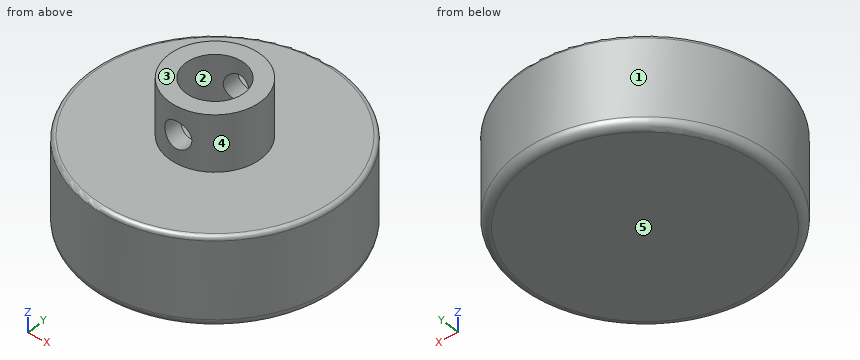
from build123d import *

# Parameters (mm, degrees)
F2_R     = 6.5
F3_DEPTH = 30


with BuildPart() as f1:
    # F0 (on Front) → F1 (revolve)
    with BuildSketch(Plane.XZ):
        with BuildLine():
            Line((-14.1, 0), (-14.1, 27))
            Line((-14.1, 27), (-22.1, 27))
            Line((-22.1, 27), (-22.1, 0))
            Line((-22.1, 0), (-58.77316, 0))
            ThreePointArc((-58.77316, 0), (-60.170035, -0.568658), (-60.772566, -1.95126))
            Line((-60.772566, -1.95126), (-60.772566, -2.403001))
            Line((-60.772566, -2.403001), (-60.772566, -39))
            ThreePointArc((-60.772566, -39), (-59.600994, -41.828427), (-56.772566, -43))
            Line((-56.772566, -43), (-56.4, -43))
            Line((-56.4, -43), (0, -43))
            Line((0, -43), (0, 0))
            Line((0, 0), (-14.1, 0))
        make_face()
    revolve(axis=Axis((0, 0, -21.5), (0, 0, -1)))

    # F2 (on Front) → F3 (cut, symmetric)
    with BuildSketch(Plane.XZ):
        with Locations((0, 13.5)):
            Circle(F2_R)
    extrude(amount=F3_DEPTH, both=True, mode=Mode.SUBTRACT)


solid = f1.part
Read the model definition and answer for the solid it produces. Units are mm, in the model's axes. Face numbers are marked on the shaded views. A direction names the side the tool comes from. Round coordinates to 2 decimals unless told otherwise and drop trailing zeros. Write each loop counter-clockwise with the first axis right and the second up, starting at its lowest first coordinate (ties: lowest second). Pieces come first, ordered by that corner, then holes. Notation, with made-up numbers: M 24,54.5 L 36,54.5 A26 ccw 36,75.5 Z; hole C 47.5,-7 d6. An arc over 180 degrees is marked long. Use a Markdown table: item, result.
1) The part is cut by section A-A (x = 0). Write down the section's boundary in (y, z).
Answers follow:
| item | result |
|---|---|
| outline | M -60.77,-39 A4 ccw -56.77,-43 L 56.77,-43 A4 ccw 60.77,-39 L 60.77,-1.95 A2 ccw 58.77,0 L 22.1,0 L 22.1,7 L 14.1,7 L 14.1,0 L -14.1,0 L -14.1,7 L -22.1,7 L -22.1,0 L -58.77,0 A2 ccw -60.77,-1.95 Z; M -22.1,20 L -14.1,20 L -14.1,27 L -22.1,27 Z; M 14.1,20 L 22.1,20 L 22.1,27 L 14.1,27 Z |
2) A tool of negligible diameter and unlimited length cuts with its end or side. For the marked faces 4 and 5, from which of +Z, -Z, +X, -X, +Y, -Y can it reach the whole face along a straight path? Write none if from no direction.
Answers follow:
| item | result |
|---|---|
| face 4 | +Z |
| face 5 | -Z, +X, -X, +Y, -Y |
3) Flat-ended cylindrical pins translate along their axes: pin 1 (4 mm diameter, centred on x = 44.5, y = 16, fed in from +Z); pin 2 (10 mm diameter, centred on y = 12.5, z = -16.5, fed in from -X); pin 3 (4 mm diameter, centred on x = 3.5, z = -3, fed in from +Y). Find the tip coordinate at first contact, or state that the pin passes through.
Answers follow:
| item | result |
|---|---|
| pin 1 | stops at z = 0 |
| pin 2 | stops at x = -60.31 |
| pin 3 | stops at y = 60.75 |
4) For a pull along X with two mould halves and no side action, classify the marked faces 1, 2 and 3 as pulls with the +X half, pulls with the -X half, needs draft (parallel to the pull), parting line crosses it, or undercut.
Answers follow:
| item | result |
|---|---|
| face 1 | parting line crosses it |
| face 2 | undercut |
| face 3 | needs draft |
5) The part is cut by section B-B (z = 13.5). Write down the section's boundary in (x, y), plus the area to 3 significant figures.
Answers follow:
| item | result |
|---|---|
| outline | M -6.5,-21.12 L -6.5,-12.51 A14.1 cw -6.5,12.51 L -6.5,21.12 A22.1 ccw Z; M 6.5,-21.12 A22.1 ccw 6.5,21.12 L 6.5,12.51 A14.1 cw 6.5,-12.51 Z |
| area | 697 mm2 |
6) The part is cut by section C-C (y = 0). Write down the section's boundary in (x, z).
Answers follow:
| item | result |
|---|---|
| outline | M -60.77,-39 A4 ccw -56.77,-43 L 56.77,-43 A4 ccw 60.77,-39 L 60.77,-1.95 A2 ccw 58.77,0 L 22.1,0 L 22.1,27 L 14.1,27 L 14.1,0 L -14.1,0 L -14.1,27 L -22.1,27 L -22.1,0 L -58.77,0 A2 ccw -60.77,-1.95 Z |
7) The part is cut by section D-D (z = -30.5). Write down the section's boundary in (x, y), plus the area to 3 significant figures.
Answers follow:
| item | result |
|---|---|
| outline | C 0,0 d121.55 |
| area | 11,600 mm2 |
8) Straight lines are drawn through the part: line 1 along Z through (x, y) = (0, -18); line 2 along Z through (x, y) = (17.5, -32); line 3 along X through (y, z) = (-17, 4). For each, find the intervals that lie inside material, in ascending order. Write a range as [from, to].
Answers follow:
| item | result |
|---|---|
| line 1 | z = [-43, 7], [20, 27] |
| line 2 | z = [-43, 0] |
| line 3 | x = [-14.12, 14.12] |
